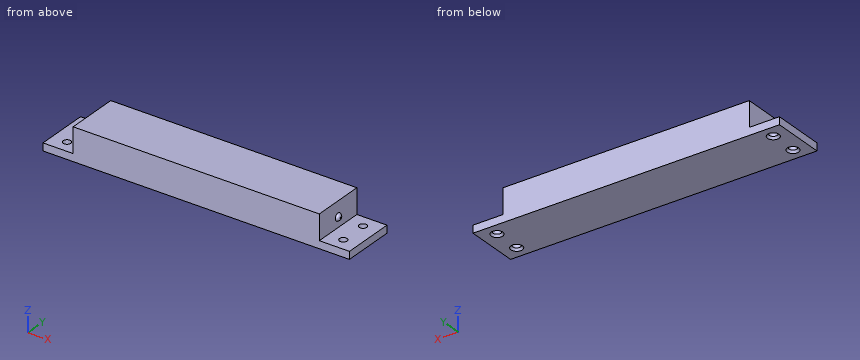
```python
from build123d import *

# Parameters (mm, degrees)
F0_W     = 155.575
F0_H     = 33.3375
F1_DEPTH = 20.6375
F0_W_2   = 19.05
F0_R     = 2.38125
F2_DEPTH = 1.5875
F3_SIZE  = 1.27
F4_R     = 2.38125
F5_DEPTH = 1.5875
F7_DEPTH = 3.175


# Not quite as in the source:
# - a fillet or chamfer that OpenCascade refuses, or shapes differently, is made with other operations: its cross-section is extruded or revolved along the edge and cut away or added


with BuildPart() as f1:
    # F0 (on Top) → F1 (new body)
    with BuildSketch(Plane.XY):
        Rectangle(F0_W, F0_H)
    extrude(amount=F1_DEPTH)

    # F0 (on Top) → F2 (join)
    with BuildSketch(Plane.XY):
        with Locations((-87.3125, 0)):
            Rectangle(F0_W_2, F0_H)
        with Locations((-87.3125, -8.73125)):
            Circle(F0_R, mode=Mode.SUBTRACT)
        with Locations((-87.3125, 8.73125)):
            Circle(F0_R, mode=Mode.SUBTRACT)
        with Locations((87.3125, 0)):
            Rectangle(F0_W_2, F0_H)
        with Locations((87.3125, -8.73125)):
            Circle(F0_R, mode=Mode.SUBTRACT)
        with Locations((87.3125, 8.73125)):
            Circle(F0_R, mode=Mode.SUBTRACT)
    extrude(amount=F2_DEPTH)

    # F3
    f3_edges = [f1.edges().sort_by_distance(p)[0] for p in [
        (-89.69375, -8.73125, 0),
        (-89.69375, 8.73125, 0),
        (84.93125, -8.73125, 0),
        (84.93125, 8.73125, 0),
    ]]
    chamfer(f3_edges, length=F3_SIZE)

    # F4 (on face) → F5 (join)
    with BuildSketch(Plane.YZ.offset(77.7875)):
        with Locations((0, 11.1125)):
            Circle(F4_R)
    extrude(amount=F5_DEPTH)

    # F6: fillet of radius 2.032 on 1 edges, made by hand

    # F6_s1 → F6_t2 (revolve, cut)
    with BuildSketch(Plane.XY.offset(11.1125)):
        with BuildLine():
            ThreePointArc((77.7875, 2.38125), (78.9292294916, 1.6684631355), (79.375, 0.3984631355))
            Line((79.375, 0.3984631355), (79.375, 2.38125))
            Line((79.375, 2.38125), (77.7875, 2.38125))
        make_face()
    revolve(axis=Axis((79.375, 0, 11.1125), (1, 0, 0)), mode=Mode.SUBTRACT)

    # F7 (add): faces of the model
    f7_faces = [f1.faces().sort_by_distance(p)[0] for p in [
        (-87.3125, 0, 1.5875),
        (87.3125, 0, 1.5875),
    ]]
    extrude(f7_faces, amount=F7_DEPTH)


solid = f1.part
```
The model under review builds one solid part; all positions refer to its coordinate system, in mm. Give positions to 0.01 mm unless a question says otherwise; leave off trailing zeros. Write each loop counter-clockwise with the first axis right and the second up, starting at its lowest first coordinate (ties: lowest second). Pieces come first, ordered by that corner, then holes. Notation, with made-up numbers: M 88.5,82 L 140.5,82 A19 cw 140.5,98 Z; hole C 60.25,27 d5. An arc over 180 degrees is marked long. Write each question's results on one line, items separated by ' | '. Start each with the question number.
1. For probe 1 along X at (y, z) = (9, 7); probe 2 along Z at (x, y) = (79, 7), list the stretches that pass through material, from the lowest coordinate up. Write a range as [from, to].
2. Insertion check: pin 1 Ø5.5 at (x, y) = (-87.31, 8.73) entering from +Z; pin 2 Ø3 at (x, y) = (87.31, -8.73) entering from -Z; pin 3 Ø4 at (y, z) = (-9, 14.5) entering from +X. Each pin has a flat end and moves straight along its axis. Give the tip position at first contact, or say it passes through.
3. We need section A-A (z = 16.5). Write out the cut boundary in (x, y).
Results found:
1) probe 1: x = [-77.79, 77.79] | probe 2: z = [0, 4.76]
2) pin 1: stops at z = 4.76 | pin 2: passes through | pin 3: stops at x = 77.79
3) outline: M -77.79,-16.67 L 77.79,-16.67 L 77.79,16.67 L -77.79,16.67 Z
